Could you check a few things on this model? Use its own coordinates, in mm. A direction names the side the tool comes from. Coordinates: 2 decimals unless noted, no trailing zeros. Loops run counter-clockwise (first coordinate to the right, second up) from the corner with the lowest first, then second, coordinate; pieces in that order, holes last.
Solid Edge part; units mm, degrees
sketch "Sketch1" plane through (0, 0, 0) normal (0, 0, 1) x (1, 0, 0)
  line L0 (-53.9742, 23.7118) -> (53.9742, 23.7118)
  line L1 (-31.7069, -8.1496) -> (31.7069, -8.1496)
  arc A0 (-31.7069, -8.1496) -> (-53.9742, 23.7118) centre (-53.9742, 0) cw
  arc A1 (53.9742, 23.7118) -> (31.7069, -8.1496) centre (53.9742, 0) cw
extrude "Protrusion1" add sketch "Sketch1" along normal mid plane 55
fillet "Round_1" radius 12 2 edges at (-31.7069, -8.1496, 0) (31.7069, -8.1496, 0)
1) We'd pull the mould along X, two halves only. Please class faces 3 (the cylindrical face through (-30.02, -9.5, 0.39)), 4 (the flat face through (1, 6, -27.5)): released by +X, released by -X, zero draft, split by the parting line, or undercut.
2) Will these pins go through, and if not, where does the flat tip stop? pin 1 (1.5 mm diameter, centred on y = 9.5, z = -2.5, fed in from +X); pin 2 (5 mm diameter, centred on y = -12, z = 5, fed in from -X); pin 3 (3 mm diameter, centred on x = -46.5, z = -0.5, fed in from -Y).
3) Imagine slicing it at B-B on x = 60.5. List the corners of the cut face in (y, z) for me, plus the area to 3 significant figures.
4) If I drill on L1, parallel to X at y = -18, z = 12.5; L2, parallel to Y at x = -20.5, z = -15; L3, parallel to X at y = -10.5, z = 14, over which ranges is the centre line in solid material (lowest first)?
5) Imagine slicing it at A-A on x = -20. List the corners of the cut face in (y, z) for me.
6) For faces 1 (the cylindrical face through (-74.6, -11.7, -0.4)), 2 (the flat face through (0, -8.15, 0)), which set-ups out of +Z, -Z, +X, -X, +Y, -Y let a thin tool reach every point of the face, with its end or its side?
Solved:
1. face 3: undercut
1. face 4: zero draft
2. pin 1: stops at x = 76.01
2. pin 2: stops at x = -75.7
2. pin 3: stops at y = -22.95
3. outline: (-22.8, -27.5) - (22.8, -27.5) - (22.8, 27.5) - (-22.8, 27.5) - close
3. area: 2,510 mm2
4. L1: x = -69.41 to -38.54, 38.54 to 69.41
4. L2: y = -8.15 to 23.71
4. L3: x = -75.23 to -31.62, 31.62 to 75.23
5. outline: (-8.15, -27.5) - (23.71, -27.5) - (23.71, 27.5) - (-8.15, 27.5) - close
6. face 1: +Z, -Z
6. face 2: +Z, -Z, -Y
